Can you work these out from the model? Positions are in its coordinate system, mm. Face numbers are marked on the shaded views. Round coordinates to 2 decimals unless told otherwise and drop trailing zeros. Loops run counter-clockwise (first coordinate to the right, second up) from the corner with the lowest first, then second, coordinate; pieces in that order, holes last. Notation, with made-up numbers: M 39,-30.5 L 98,-30.5 A31 cw 98,8.5 Z; hole C 85,83 d9. An arc over 180 degrees is marked long. Answer as CSV lines item,"result".
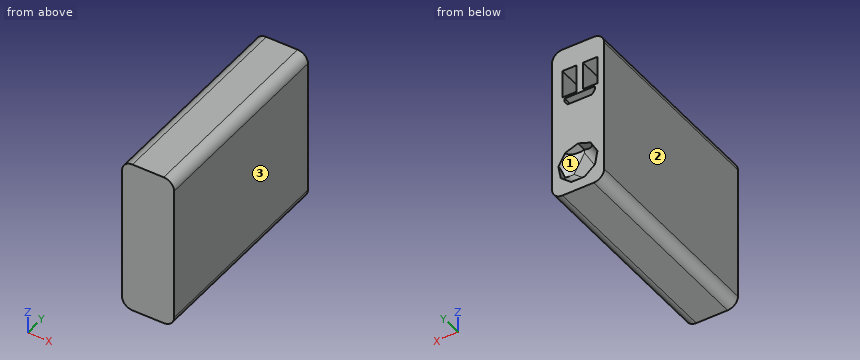
from build123d import *

# Parameters (mm, degrees)
F0_W          = 99.8685956001
F0_H          = 76.2
F1_DEPTH      = 25.4
F2_R          = 5.08
F3_R          = 5.08
F4_R          = 5.08
F5_R          = 5.08
F6_W          = 7
F6_H          = 13.8
F7_DEPTH      = 15
F8_W          = 14.7339338437
F8_H          = 1.7859311774
F9_DEPTH      = 15
F11_DEPTH     = 5
F12_T4_DEPTH  = 32.018367851
F12_T10_DEPTH = 32.018367851
F12_T17_DEPTH = 32.018367851
F12_T23_DEPTH = 32.018367851


# Not quite as in the source:
# - a fillet or chamfer that OpenCascade refuses, or shapes differently, is made with other operations: its cross-section is extruded or revolved along the edge and cut away or added


with BuildPart() as f1:
    # F0 (on Right) → F1 (new body)
    with BuildSketch(Plane.YZ):
        Rectangle(F0_W, F0_H)
    extrude(amount=F1_DEPTH)

    # F2
    f2_edges = [f1.edges().sort_by_distance(p)[0] for p in [
        (25.4, 0, 38.1),
    ]]
    fillet(f2_edges, radius=F2_R)

    # F3
    f3_edges = [f1.edges().sort_by_distance(p)[0] for p in [
        (0, 0, 38.1),
    ]]
    fillet(f3_edges, radius=F3_R)

    # F4
    f4_edges = [f1.edges().sort_by_distance(p)[0] for p in [
        (25.4, 0, -38.1),
    ]]
    fillet(f4_edges, radius=F4_R)

    # F5
    f5_edges = [f1.edges().sort_by_distance(p)[0] for p in [
        (0, 0, -38.1),
    ]]
    fillet(f5_edges, radius=F5_R)

    # F6 (on face) → F7 (cut)
    with BuildSketch(Plane(origin=(0, 49.9342978001, 0), x_dir=(-1, 0, 0), z_dir=(0, 1, 0))):
        with Locations((-6.8276954116, 20.0042553112)):
            Rectangle(F6_W, F6_H)
        with Locations((-16.8951429576, 20.0042553112)):
            Rectangle(F6_W, F6_H)
    extrude(amount=-F7_DEPTH, mode=Mode.SUBTRACT)

    # F8 (on face) → F9 (cut)
    with BuildSketch(Plane(origin=(0, 49.9342978001, 0), x_dir=(-1, 0, 0), z_dir=(0, 1, 0))):
        with Locations((-11.9025348686, 11.1820721067)):
            Rectangle(F8_W, F8_H)
        Polygon((-4.5355679467, 10.289106518), (-19.2695017904, 10.289106518), (-17.8024861962, 8.3756083623), (-5.9387991205, 8.3756083623), align=None)
    extrude(amount=-F9_DEPTH, mode=Mode.SUBTRACT)

    # F10 (on face) → F11 (cut)
    with BuildSketch(Plane(origin=(0, 49.9342978001, 0), x_dir=(-1, 0, 0), z_dir=(0, 1, 0))):
        Polygon((-16.0813947992, -32.9593643546), (-9.4630269482, -32.9593643546), (-4.3930630334, -28.7051595036), (-3.2437955169, -22.1873395316), (-6.5529794424, -16.4556648411), (-12.7722108737, -14.1920497201), (-18.9914423049, -16.4556648411), (-22.3006262304, -22.1873395316), (-21.151358714, -28.7051595036), align=None)
    extrude(amount=-F11_DEPTH, mode=Mode.SUBTRACT)

    # F12: fillet of radius 5.08 on 4 edges, made by hand


with BuildPart() as f12_tool2:
    # F12_s3 → F12_t4 (new body)
    with BuildSketch(Plane(origin=(5.5233724705, 0, -9.566761748), x_dir=(0, 1, 0), z_dir=(0.5, 0, -0.8660254038))):
        with BuildLine():
            ThreePointArc((50.0142978001, 8.21923907), (46.4221953516, 6.7313415185), (44.9342978001, 3.13923907))
            Line((44.9342978001, 3.13923907), (44.9342978001, 8.21923907))
            Line((44.9342978001, 8.21923907), (50.0142978001, 8.21923907))
        make_face()
    extrude(amount=F12_T4_DEPTH)

    split(bisect_by=Plane.XZ.offset(-49.9342978001), keep=Keep.TOP)

    split(bisect_by=Plane(origin=(25.4224385924, 0, -4.4826618392), x_dir=(0, 1, 0), z_dir=(-0.984807753, 0, 0.1736481777)), keep=Keep.TOP)


with BuildPart() as f1_1:
    add(f1.part)

    # F12_t1: union F12_tool2
    add(f12_tool2.part)


with BuildPart() as f12_tool8:
    # F12_s9 → F12_t10 (new body)
    with BuildSketch(Plane(origin=(31.5112153695, 0, -26.4410491945), x_dir=(0, 1, 0), z_dir=(-0.7660444431, 0, 0.6427876097))):
        with BuildLine():
            ThreePointArc((50.0142978001, 19.1656214402), (46.4221953516, 17.6777238886), (44.9342978001, 14.0856214402))
            Line((44.9342978001, 14.0856214402), (44.9342978001, 19.1656214402))
            Line((44.9342978001, 19.1656214402), (50.0142978001, 19.1656214402))
        make_face()
    extrude(amount=F12_T10_DEPTH)

    split(bisect_by=Plane.XZ.offset(-49.9342978001), keep=Keep.TOP)

    split(bisect_by=Plane(origin=(-0.6482754096, 0, -0.1143084456), x_dir=(0, 1, 0), z_dir=(0.984807753, 0, 0.1736481777)), keep=Keep.TOP)

    split(bisect_by=Plane.XY.offset(-32.9593643546), keep=Keep.TOP)


with BuildPart() as f1_2:
    add(f1_1.part)

    # F12_t7: union F12_tool8
    add(f12_tool8.part)


with BuildPart() as f12_tool15:
    # F12_s16 → F12_t17 (new body)
    with BuildSketch(Plane(origin=(-15.1464509592, 0, -26.2344226156), x_dir=(0, 1, 0), z_dir=(0.5, 0, 0.8660254038))):
        with BuildLine():
            ThreePointArc((50.0142978001, -13.9028790881), (46.4221953516, -15.3907766397), (44.9342978001, -18.9828790881))
            Line((44.9342978001, -18.9828790881), (44.9342978001, -13.9028790881))
            Line((44.9342978001, -13.9028790881), (50.0142978001, -13.9028790881))
        make_face()
    extrude(amount=F12_T17_DEPTH)

    split(bisect_by=Plane.XZ.offset(-49.9342978001), keep=Keep.TOP)

    split(bisect_by=Plane(origin=(-12.3194239937, 0, -14.6817178032), x_dir=(0, 1, 0), z_dir=(0.6427876097, 0, 0.7660444431)), keep=Keep.TOP)


with BuildPart() as f1_3:
    add(f1_2.part)

    # F12_t14: union F12_tool15
    add(f12_tool15.part)


with BuildPart() as f12_tool21:
    # F12_s22 → F12_t23 (new body)
    with BuildSketch(Plane(origin=(8.0063594172, 0, 6.7181332341), x_dir=(0, 1, 0), z_dir=(-0.7660444431, 0, -0.6427876097))):
        with BuildLine():
            ThreePointArc((50.0142978001, 35.585259236), (46.4221953516, 34.0973616844), (44.9342978001, 30.505259236))
            Line((44.9342978001, 30.505259236), (44.9342978001, 35.585259236))
            Line((44.9342978001, 35.585259236), (50.0142978001, 35.585259236))
        make_face()
    extrude(amount=F12_T23_DEPTH)

    split(bisect_by=Plane.XZ.offset(-49.9342978001), keep=Keep.TOP)

    split(bisect_by=Plane(origin=(7.1180698344, 0, 4.109619535), x_dir=(0, 1, 0), z_dir=(-0.8660254038, 0, -0.5)), keep=Keep.TOP)

    split(bisect_by=Plane.XY.offset(-32.9593643546), keep=Keep.TOP)


with BuildPart() as f1_4:
    add(f1_3.part)

    # F12_t20: union F12_tool21
    add(f12_tool21.part)


solid = f1_4.part
Item 1: We'd pull the mould along X, two halves only. Please class the marked faces 1, 2 and 3: released by +X, released by -X, zero draft, split by the parting line, or undercut.
Output:
face 1,"undercut"
face 2,"released by -X"
face 3,"released by +X"
Item 2: Will these pins go through, and if not, where does the flat tip stop? pin 1 (1.1 mm diameter, centred on x = 14, z = 9.5, fed in from +Y); pin 2 (5 mm diameter, centred on x = 14, z = -25.5, fed in from +Y).
Output:
pin 1,"stops at y = 34.93"
pin 2,"stops at y = 44.96"
Item 3: If we section it at A-A on y = 42: Write out the boundary of the cut face in (x, z).
Output:
outline,"M 0,-33.02 A5.08 ccw 5.08,-38.1 L 20.32,-38.1 A5.08 ccw 25.4,-33.02 L 25.4,33.02 A5.08 ccw 20.32,38.1 L 5.08,38.1 A5.08 ccw 0,33.02 Z; hole M 3.33,13.1 L 10.33,13.1 L 10.33,26.9 L 3.33,26.9 Z; hole M 4.54,10.29 L 5.94,8.38 L 17.8,8.38 L 19.27,10.29 L 19.27,12.08 L 4.54,12.08 Z; hole M 13.4,13.1 L 20.4,13.1 L 20.4,26.9 L 13.4,26.9 Z"
Item 4: If I drill on line 1 along X through (y, z) = (40.5, 23); line 2 along Y through (x, z) = (5.75, 26.5); line 3 along Y through (x, z) = (11.5, -16.5), over which ranges is the centre line in solid material (lowest first)? Write a range as from..to.
Output:
line 1,"x = 0..3.33, 10.33..13.4, 20.4..25.4"
line 2,"y = -49.93..34.93"
line 3,"y = -49.93..44.99"
